The drawing under review shows one solid part. Ordinate dimensions are in mm from its lowest x, y, z. Coordinates: 2 decimals unless noted, no trailing zeros. Order: outer loops, then holes, each group sorted by start corner. A loop starts at its lowest first (then second) coordinate and runs counter-clockwise, first axis right, second up. Notation, with made-up numbers: M 25.25,78 L 78.25,78 A27 cw 78.25,108 Z; hole C 41,-20 d2. An arc over 180 degrees is marked long. Answer as a JSON object with one key per item and string values.
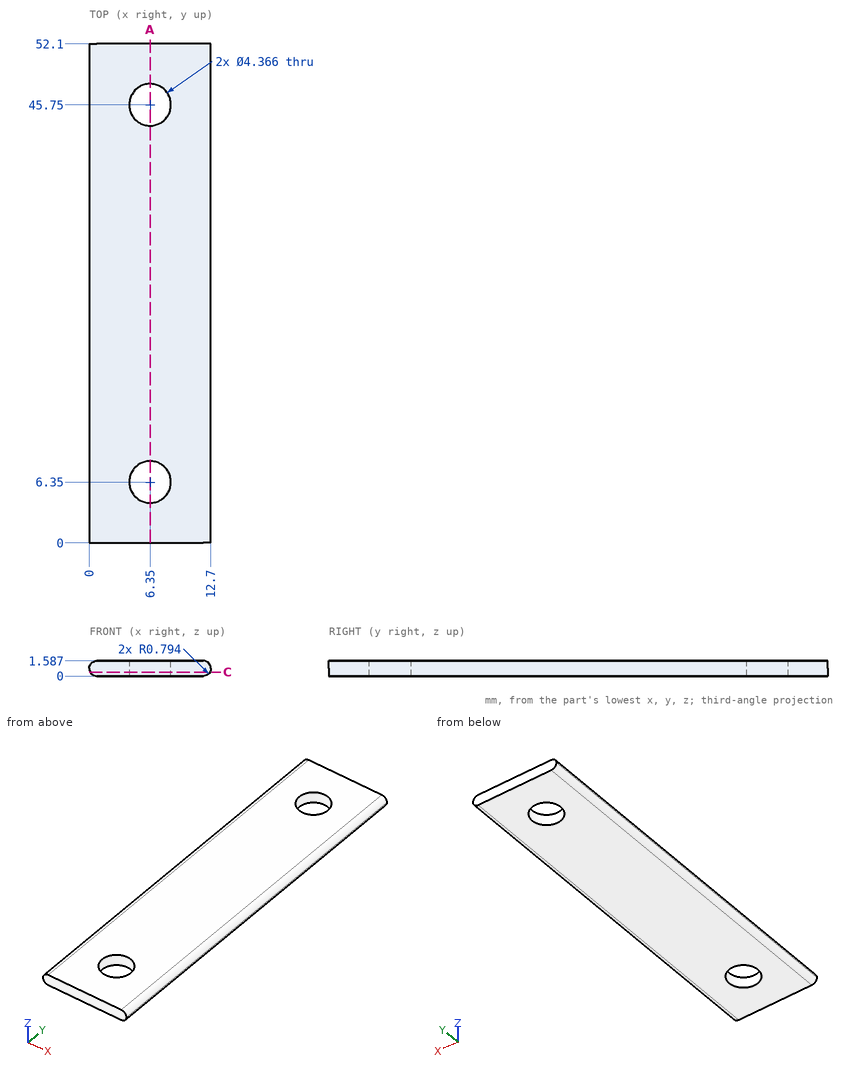
1) Add section C-C (z = 0.4). Count the separate pieces of the cut face and the enclosed holes in it, and give its area (3 significant figures).
Taken from the geometry:
{"separate pieces": "1", "enclosed holes": "2", "area": "621 mm2"}
2) To check wall thickness, follow L1, parallel to Y at x = 6.35, z = 1.35; L2, parallel to Y at x = 7, z = 1.3 (1 decimal); L3, parallel to X at y = 8, z = 0.4 (1 decimal). State the ranges of each line that lie inside material, in increasing order.
Taken from the geometry:
{"L1": "y = 0 to 4.17, 8.53 to 43.57, 47.93 to 52.1", "L2": "y = 0 to 4.3, 8.4 to 43.7, 47.8 to 52.1", "L3": "x = 0.1 to 4.9, 7.8 to 12.6"}
3) Insertion check: pin 1 Ø3.5 at (x, y) = (6.35, 45.75) entering from -Z. The pin has a flat end and moves straight along its axis. Give the tip position at first contact, or say it passes through.
Taken from the geometry:
{"pin 1": "passes through"}
4) Add section A-A (x = 6.35). State the section outline as (y, z) points.
Taken from the geometry:
{"outline": "M 0,0 L 4.17,0 L 4.17,1.59 L 0,1.59 Z; M 8.53,0 L 43.57,0 L 43.57,1.59 L 8.53,1.59 Z; M 47.93,0 L 52.1,0 L 52.1,1.59 L 47.93,1.59 Z"}
